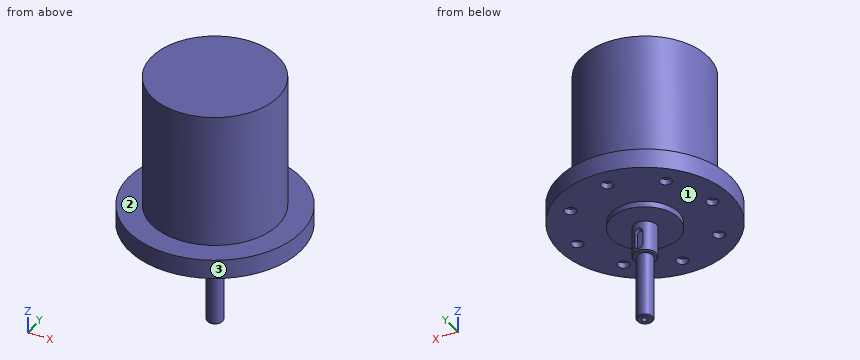
from build123d import *

# Parameters (mm, degrees)
CUT_EXTRUDE1_DEPTH = 2.5
CHAMFER1_SIZE      = 0.5
SKETCH7_R          = 3
CUT_EXTRUDE4_DEPTH = 3
SKETCH8_R          = 1.5
CUT_EXTRUDE5_DEPTH = 5
CHAMFER2_SIZE      = 0.5


with BuildPart() as part:
    # Sketch1 → Revolve1 (revolve)
    with BuildSketch(Plane(origin=(0, 0, 0), x_dir=(0, 0, -1), z_dir=(1, 0, 0)), mode=Mode.PRIVATE) as revolve1_sk:
        Polygon((-67.783857366, 0), (65.216142634, 0), (65.216142634, 4), (31.216142634, 4), (31.216142634, 6), (15.216142634, 6), (15.216142634, 17.5), (12.216142634, 17.5), (12.216142634, 45), (2.216142634, 45), (2.216142634, 33), (-67.783857366, 33), align=None)
    revolve(revolve1_sk.sketch.rotate(Axis((0, 0, 67.783857366), (0, 0, -1)), 180), axis=Axis((0, 0, 67.783857366), (0, 0, -1)))

    # Sketch2 → Cut-Extrude1 (cut)
    with BuildSketch(Plane(origin=(0, 6, 0), x_dir=(1, 0, 0), z_dir=(0, 1, 0))):
        with BuildLine():
            Line((-2.025, 20.732267436), (-2.025, 27.682267436))
            ThreePointArc((-2.025, 27.682267436), (0, 29.707267436), (2.025, 27.682267436))
            Line((2.025, 27.682267436), (2.025, 20.732267436))
            ThreePointArc((2.025, 20.732267436), (0, 18.707267436), (-2.025, 20.732267436))
        make_face()
    extrude(amount=-CUT_EXTRUDE1_DEPTH, mode=Mode.SUBTRACT)

    # Chamfer1
    chamfer1_edges = [part.edges().sort_by_distance(p)[0] for p in [
        (0, 6, -31.216142634),
    ]]
    chamfer(chamfer1_edges, length=CHAMFER1_SIZE)

    # Sketch7 → Cut-Extrude4 (cut)
    with BuildSketch(Plane(origin=(0, 0, -12.216142634), x_dir=(-1, 0, 0), z_dir=(0, 0, -1))):
        with Locations(Location((0, 35, 0), (0, 0, 90))):
            Circle(SKETCH7_R)
        with Locations(Location((24.748737342, 24.748737342, 0), (0, 0, 90))):
            Circle(SKETCH7_R)
        with Locations(Location((35, 0, 0), (0, 0, 90))):
            Circle(SKETCH7_R)
        with Locations(Location((24.748737342, -24.748737342, 0), (0, 0, 90))):
            Circle(SKETCH7_R)
        with Locations(Location((0, -35, 0), (0, 0, 90))):
            Circle(SKETCH7_R)
        with Locations(Location((-24.748737342, -24.748737342, 0), (0, 0, 90))):
            Circle(SKETCH7_R)
        with Locations(Location((-35, 0, 0), (0, 0, 90))):
            Circle(SKETCH7_R)
        with Locations(Location((-24.748737342, 24.748737342, 0), (0, 0, 90))):
            Circle(SKETCH7_R)
    extrude(amount=-CUT_EXTRUDE4_DEPTH, mode=Mode.SUBTRACT)

    # Sketch8 → Cut-Extrude5 (cut)
    with BuildSketch(Plane(origin=(0, 0, -65.216142634), x_dir=(-1, 0, 0), z_dir=(0, 0, -1))):
        with Locations(Location((0, 0, 0), (0, 0, 90))):
            Circle(SKETCH8_R)
    extrude(amount=-CUT_EXTRUDE5_DEPTH, mode=Mode.SUBTRACT)

    # Chamfer2
    chamfer2_edges = [part.edges().sort_by_distance(p)[0] for p in [
        (0, 4, -65.216142634),
    ]]
    chamfer(chamfer2_edges, length=CHAMFER2_SIZE)


solid = part.part
The model under review builds one solid part; all positions refer to its coordinate system, in mm. Face numbers are marked on the shaded views. A direction names the side the tool comes from. Give positions to 0.01 mm unless a question says otherwise; leave off trailing zeros. Order: outer loops, then holes, each group sorted by start corner. A loop starts at its lowest first (then second) coordinate and runs counter-clockwise, first axis right, second up. Notation, with made-up numbers: M 27.25,74.25 L 37.25,74.25 A36 cw 37.25,110.25 Z; hole C 47.5,-17.5 d10. An arc over 180 degrees is marked long. Answer in a Markdown table with one row per item. Add a question column.
1. Add section A-A on x = 20. State the section outline as (y, z) points.
2. Machinability: for the marked faces 1, 2 and 3, which of the approach directions +Z, -Z, +X, -X, +Y, -Y give a long, thin tool a straight path to every point of the face, cutting with its end or side? Answer none if there is none.
3. Add section C-C on z = 6.5. State the section outline as (x, y) points, plus the area to 3 significant figures.
4. To check wall thickness, follow line 1 along X through (y, z) = (0, -11); line 2 along Z through (x, y) = (-14, -11.5); line 3 along X through (y, z) = (0, -61.3). State the ranges of each line that lie inside material, in increasing order.
5. Add section D-D on x = 10. State the section outline as (y, z) points.
6. Add section B-B on y = -35. State the section outline as (x, z) points, plus the area to 3 significant figures.
7. For pin 1 Ø1.8 at (x, y) = (25.5, 26) entering from -Z; pin 2 Ø6 at (x, y) = (-32.5, -4.5) entering from -Z; pin 3 Ø3 at (x, z) = (1, -24) entering from +Y; pin 4 Ø12 at (y, z) = (-32, -21) entering from +X, all flat-tipped, find the tip position at first contact; note any pin that passes through.
The answers:
| question | item | result |
|---|---|---|
| 1 | outline | M -40.31,-12.22 L 40.31,-12.22 L 40.31,-2.22 L 26.25,-2.22 L 26.25,67.78 L -26.25,67.78 L -26.25,-2.22 L -40.31,-2.22 Z |
| 2 | face 1 | -Z |
| 2 | face 2 | +Z |
| 2 | face 3 | +Z, -Z |
| 3 | outline | C 0,0 d66 |
| 3 | area | 3,420 mm2 |
| 4 | line 1 | -45 to -38, -32 to 32, 38 to 45 |
| 4 | line 2 | -12.22 to 67.78 |
| 4 | line 3 | -4 to -1.5, 1.5 to 4 |
| 5 | outline | M -43.87,-12.22 L -14.36,-12.22 L -14.36,-15.22 L 14.36,-15.22 L 14.36,-12.22 L 43.87,-12.22 L 43.87,-2.22 L 31.45,-2.22 L 31.45,67.78 L -31.45,67.78 L -31.45,-2.22 L -43.87,-2.22 Z |
| 6 | outline | M -28.28,-12.22 L -3,-12.22 L -3,-9.22 L 3,-9.22 L 3,-12.22 L 28.28,-12.22 L 28.28,-2.22 L -28.28,-2.22 Z |
| 6 | area | 548 mm2 |
| 7 | pin 1 | z = -9.22 |
| 7 | pin 2 | z = -12.22 |
| 7 | pin 3 | y = 5.65 |
| 7 | pin 4 | through |
